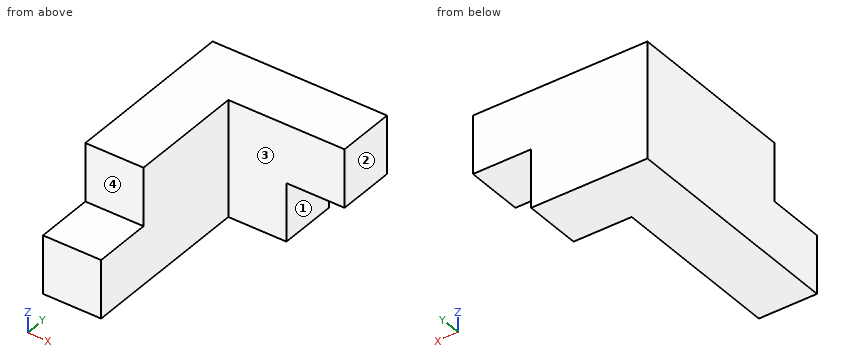
```python
from build123d import *

# Parameters (mm, degrees)
F0_W     = 101.6
F0_H     = 50.8
F1_DEPTH = 25.4
F2_W     = 25.4
F2_H     = 25.4
F3_DEPTH = 25.4
F4_W     = 25.4
F4_H     = 50.8
F5_DEPTH = 25.4
F6_W     = 25.4
F6_H     = 25.4
F7_DEPTH = 25.4


with BuildPart() as f1:
    # F0 (on Right) → F1 (new body)
    with BuildSketch(Plane.YZ):
        with Locations((50.8, 25.4)):
            Rectangle(F0_W, F0_H)
    extrude(amount=F1_DEPTH)

    # F2 (on face) → F3 (cut)
    with BuildSketch(Plane.YZ.offset(25.4)):
        with Locations((12.7, 38.1)):
            Rectangle(F2_W, F2_H)
    extrude(amount=-F3_DEPTH, mode=Mode.SUBTRACT)

    # F4 (on face) → F5 (join)
    with BuildSketch(Plane.YZ.offset(25.4)):
        with Locations((88.9, 25.4)):
            Rectangle(F4_W, F4_H)
    extrude(amount=F5_DEPTH)

    # F6 (on face) → F7 (join)
    with BuildSketch(Plane.YZ.offset(50.8)):
        with Locations((88.9, 38.1)):
            Rectangle(F6_W, F6_H)
    extrude(amount=F7_DEPTH)


solid = f1.part
```
Check sheet for the modelled part. Datum: model origin and axes. Units: mm. Face numbers are marked on the shaded views. A direction names the side the tool comes from. Round coordinates to 2 decimals unless told otherwise and drop trailing zeros. Order: outer loops, then holes, each group sorted by start corner. A loop starts at its lowest first (then second) coordinate and runs counter-clockwise, first axis right, second up. Notation, with made-up numbers: (-18, -3) - (12, -3) arc R23 ccw to (12, 12) - close; hole circle Ø9 at (-17.5, -31). An arc over 180 degrees is marked (long way). Write item = value, one per line.
Q1. Thickness scan on line 1 along Y through (x, z) = (29, 26.5); line 2 along X through (y, z) = (49.5, 4). Record the ranges inside material, lowest first.
Computed:
line_1 = 76.2 to 101.6
line_2 = 0 to 25.4
Q2. Section check A-A (z = 40). Record the boundary of the cut face in (x, y), and give its area (3 significant figures).
Computed:
outline = (0, 25.4) - (25.4, 25.4) - (25.4, 76.2) - (76.2, 76.2) - (76.2, 101.6) - (0, 101.6) - close
area = 3,230 mm^2
Q3. Section check D-D (y = 71.5). Record the boundary of the cut face in (x, z), and give its area (3 significant figures).
Computed:
outline = (0, 0) - (25.4, 0) - (25.4, 50.8) - (0, 50.8) - close
area = 1,290 mm^2
Q4. Tool access check on the marked faces 1, 2, 3 and 4. Record the directions out of +Z, -Z, +X, -X, +Y, -Y that give a thin tool (end or side, any length) a straight path to the whole face; none if there is none.
Computed:
face_1 = -Z, +X, +Y, -Y
face_2 = +Z, -Z, +X, +Y, -Y
face_3 = +Z, -Z, +X, -Y
face_4 = +Z, +X, -X, -Y
Q5. Section check B-B (y = 91). Record the boundary of the cut face in (x, z).
Computed:
outline = (0, 0) - (50.8, 0) - (50.8, 25.4) - (76.2, 25.4) - (76.2, 50.8) - (0, 50.8) - close
Q6. Go/stop test with flat-tipped pins: pin 1 (6 mm diameter, centred on y = 88.5, z = 20, fed in from +X); pin 2 (1 mm diameter, centred on y = 53.5, z = 9.5, fed in from +X); pin 3 (15 mm diameter, centred on x = 59, z = 37.5, fed in from -Y). Record where each tip stops, or that it passes through.
Computed:
pin_1 = 50.8
pin_2 = 25.4
pin_3 = 76.2
Q7. Section check C-C (x = 56.5). Record the boundary of the cut face in (y, z).
Computed:
outline = (76.2, 25.4) - (101.6, 25.4) - (101.6, 50.8) - (76.2, 50.8) - close
